Here's the drawing with two shaded views (mm, measured from the low corner). I have some questions. Coordinates: 2 decimals unless noted, no trailing zeros. Order: outer loops, then holes, each group sorted by start corner. A loop starts at its lowest first (then second) coordinate and runs counter-clockwise, first axis right, second up. Notation, with made-up numbers: (14.25, 80) -> (59.25, 80) arc R19 cw to (59.25, 89) -> close; hole circle Ø2 at (-22.5, 51.5). An arc over 180 degrees is marked (long way). Answer as a JSON object with one key per item and string values. Group by question number.
(1) For pin 1 (1.9 mm diameter, centred on x = 82, y = 4, fed in from +Z); pin 2 (1.9 mm diameter, centred on x = 70, y = 2.5, fed in from -Z), each with a flat end and sliding along its axis, tell me the tip position at first contact or that it passes through.
(2) I want a section at B-B, the plane x = 61. List the corners of the cut face in (y, z) for me.
(3) I want a section at A-A, the plane y = 5. List the corners of the cut face in (x, z) for me.
(4) I need wall thicknesses on line 1 (Z direction, x = 59, y = 1.25). Which ranges of the line are inside material? Lowest first, please.
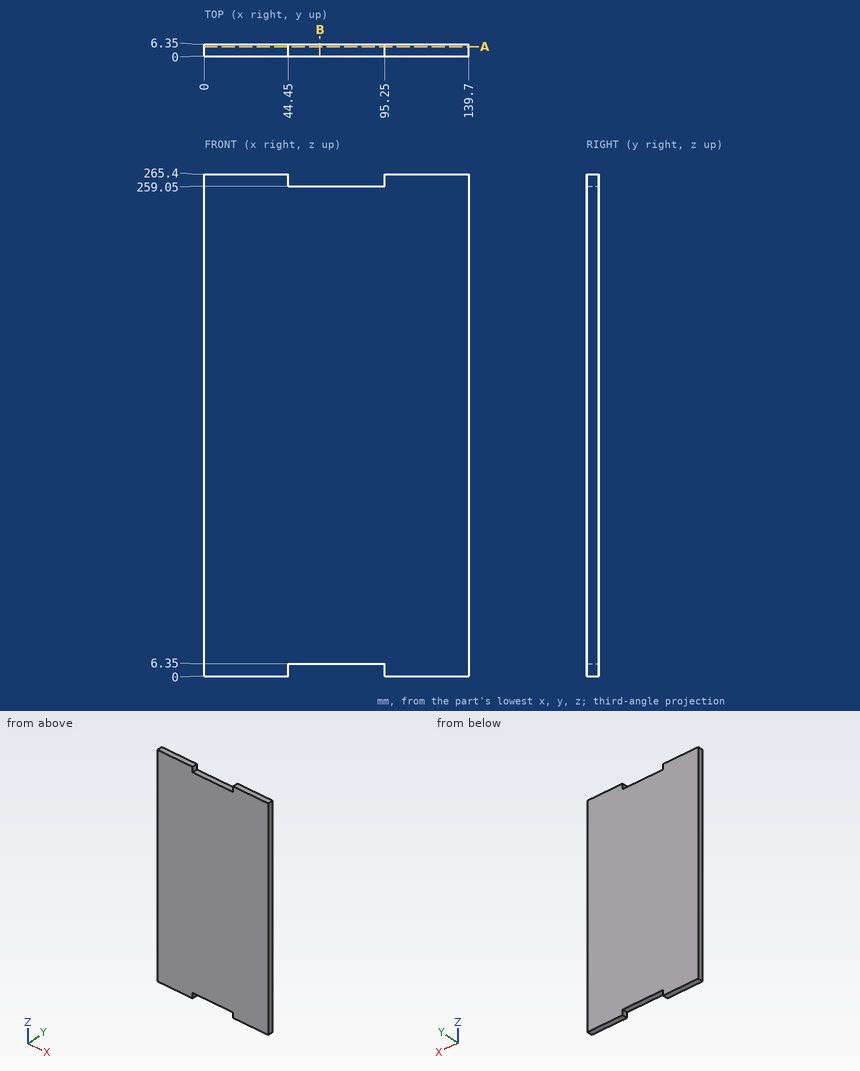
Computed values:
{
 "1": {"pin 1": "stops at z = 259.05", "pin 2": "stops at z = 6.35"},
 "2": {"outline": "(0, 6.35) -> (6.35, 6.35) -> (6.35, 259.05) -> (0, 259.05) -> close"},
 "3": {"outline": "(0, 0) -> (44.45, 0) -> (44.45, 6.35) -> (95.25, 6.35) -> (95.25, 0) -> (139.7, 0) -> (139.7, 265.4) -> (95.25, 265.4) -> (95.25, 259.05) -> (44.45, 259.05) -> (44.45, 265.4) -> (0, 265.4) -> close"},
 "4": {"line 1": "z = 6.35 to 259.05"}
}
